Read the model definition and answer for the solid it produces. Units are mm, in the model's axes. A direction names the side the tool comes from. Round coordinates to 2 decimals unless told otherwise and drop trailing zeros. Loops run counter-clockwise (first coordinate to the right, second up) from the corner with the lowest first, then second, coordinate; pieces in that order, holes last. Notation, with made-up numbers: (-40, 88) - (-29, 88) arc R32 ccw to (-29, 124) - close; hole circle Ø11 at (72.5, 28.25). An arc over 180 degrees is marked (long way). Answer as CSV lines item,"result".
Autodesk Inventor part; units mm, degrees
ref_plane "YZ Plane" through (0, 0, 0) normal (1, 0, 0) x (0, 1, 0)
ref_plane "XZ Plane" through (0, 0, 0) normal (0, 1, 0) x (-1, 0, 0)
ref_plane "XY Plane" through (0, 0, 0) normal (0, 0, 1) x (1, 0, 0)
sketch "Boceto1" plane through (0, 0, 0) normal (0, 1, 0) x (-1, 0, 0)
  line L0 (-3, 3) -> (3, 3)
  line L1 (3, 3) -> (3, -3)
  line L2 (3, -3) -> (-3, -3)
  line L3 (-3, -3) -> (-3, 3)
  line L4 (-3, 3) -> (3, -3) construction
  line L5 (3, 3) -> (-3, -3) construction
  point P0 (0, 0)
  dimension "d0" = 6
  dimension "d1" = 6
extrude "Extrusión1" add sketch "Boceto1" along normal blind 5
sketch "Boceto2" plane through (0, 5, 0) normal (0, 1, 0) x (1, 0, 0)
  circle A0 centre (0, 0) radius 2
  dimension "d4" = 4
extrude "Extrusión2" add sketch "Boceto2" along normal blind 7
sketch "Boceto3" plane through (0, 12, 0) normal (0, 1, 0) x (1, 0, 0)
  circle A0 centre (0, 0) radius 0.25
  dimension "d7" = 0.5
extrude "Extrusión3" add sketch "Boceto3" along normal blind 3
properties part number "Herramienta" material "Hierro, fundido"
1) A cutting plane is placed at C-C, the plane y = 6. Determine the outline of the cut face in (x, z).
Entries:
outline,"circle Ø4 at (0, 0)"
2) A cutting plane is placed at D-D, the plane x = -1.75. Determine the outline of the cut face in (y, z), plus the area to 3 significant figures.
Entries:
outline,"(0, -3) - (5, -3) - (5, -0.97) - (12, -0.97) - (12, 0.97) - (5, 0.97) - (5, 3) - (0, 3) - close"
area,"43.6 mm^2"
3) Find the intervals of material crossed by line 1 (Z direction, x = 0, y = 9.5); line 2 (Y direction, x = 1.85, z = -2); line 3 (Y direction, x = -1.35, z = 0.7), in increasing order.
Entries:
line 1,"z = -2 to 2"
line 2,"y = 0 to 5"
line 3,"y = 0 to 12"
4) A tool of negligible diameter and unlimited length cuts with its end or side. For faces 1 (the face through (-3, 2, 0)), 2 (the face through (0, 8, -2)), from which of +Z, -Z, +X, -X, +Y, -Y can it reach the whole face along a straight path? Write none if from no direction.
Entries:
face 1,"+Z, -Z, -X, +Y, -Y"
face 2,"+Y"
5) A cutting plane is placed at B-B, the plane x = 0. Determine the outline of the cut face in (y, z).
Entries:
outline,"(0, -3) - (5, -3) - (5, -2) - (12, -2) - (12, -0.25) - (15, -0.25) - (15, 0.25) - (12, 0.25) - (12, 2) - (5, 2) - (5, 3) - (0, 3) - close"
6) A cutting plane is placed at A-A, the plane z = 0. Determine the outline of the cut face in (x, y).
Entries:
outline,"(-3, 0) - (3, 0) - (3, 5) - (2, 5) - (2, 12) - (0.25, 12) - (0.25, 15) - (-0.25, 15) - (-0.25, 12) - (-2, 12) - (-2, 5) - (-3, 5) - close"
